from build123d import *

# Parameters (mm, degrees)
F2_W      = 22
F2_H      = 45.6
F2_R      = 1.7
F3_DEPTH  = 4
F4_R      = 5
F5_R      = 3.99999
F6_DEPTH  = 3
F8_R      = 9
F9_DEPTH  = 12
F10_R     = 2.85
F11_DEPTH = 8
F12_R     = 2.15
F13_DEPTH = 8
F13_TAPER = -0.5
F14_SIZE2 = 4
F14_SIZE  = 2


# Not quite as in the source:
# - a fillet or chamfer is up to 0.001 mm smaller than in the source, because OpenCascade refuses the exact size
# - a feature names something its author has since deleted; it is built from what else it names


with BuildPart() as f3:
    # F2 (on Top) → F3 (new body)
    with BuildSketch(Plane.XY):
        Rectangle(F2_W, F2_H)
        Polygon((3.3486315613, -16.9), (1.6743157806, -19.8), (-1.6743157806, -19.8), (-3.3486315613, -16.9), (-1.6743157806, -14), (1.6743157806, -14), align=None, mode=Mode.SUBTRACT)
        Circle(F2_R, mode=Mode.SUBTRACT)
        Polygon((1.6743157806, 19.8), (3.3486315613, 16.9), (1.6743157806, 14), (-1.6743157806, 14), (-3.3486315613, 16.9), (-1.6743157806, 19.8), align=None, mode=Mode.SUBTRACT)
        Polygon((1.6743157806, 14), (3.3486315613, 16.9), (1.6743157806, 19.8), (-1.6743157806, 19.8), (-3.3486315613, 16.9), (-1.6743157806, 14), align=None)
        with Locations((0, 16.9)):
            Circle(F2_R, mode=Mode.SUBTRACT)
        Circle(F2_R)
        Polygon((-1.6743157806, -19.8), (1.6743157806, -19.8), (3.3486315613, -16.9), (1.6743157806, -14), (-1.6743157806, -14), (-3.3486315613, -16.9), align=None)
        with Locations((0, -16.9)):
            Circle(F2_R, mode=Mode.SUBTRACT)
    extrude(amount=-F3_DEPTH)

    # F4
    f4_edges = [f3.edges().sort_by_distance(p)[0] for p in [
        (-11, 22.8, -2),
        (11, 22.8, -2),
        (11, -22.8, -2),
        (-11, -22.8, -2),
    ]]
    fillet(f4_edges, radius=F4_R)

    # F5 (radius 4 in the source; OpenCascade refuses exactly that, so slightly less here)
    f5_edges = [f3.edges().sort_by_distance(p)[0] for p in [
        (-11, 0, 0),
        (0, -22.8, 0),
        (-9.535534, -21.335534, 0),
        (9.535534, -21.335534, 0),
        (11, 0, 0),
        (9.535534, 21.335534, 0),
        (0, 22.8, 0),
        (-9.535534, 21.335534, 0),
    ]]
    fillet(f5_edges, radius=F5_R)

    # F2 (on Top) → F6 (cut)
    with BuildSketch(Plane.XY):
        Polygon((1.6743157806, 14), (3.3486315613, 16.9), (1.6743157806, 19.8), (-1.6743157806, 19.8), (-3.3486315613, 16.9), (-1.6743157806, 14), align=None)
        with Locations((0, 16.9)):
            Circle(F2_R, mode=Mode.SUBTRACT)
        Polygon((-1.6743157806, -19.8), (1.6743157806, -19.8), (3.3486315613, -16.9), (1.6743157806, -14), (-1.6743157806, -14), (-3.3486315613, -16.9), align=None)
        with Locations((0, -16.9)):
            Circle(F2_R, mode=Mode.SUBTRACT)
    extrude(amount=-F6_DEPTH, mode=Mode.SUBTRACT)

    # F8 (on line) → F9 (join)
    with BuildSketch(Plane.XY):
        Circle(F8_R)
    extrude(amount=F9_DEPTH)

    # F10 (on face) → F11 (cut)
    with BuildSketch(Plane.XY.offset(12)):
        Circle(F10_R)
    extrude(amount=-F11_DEPTH, mode=Mode.SUBTRACT)

    # F12 (on face) → F13 (cut, through all)
    with BuildSketch(Plane.XY.offset(4)):
        Circle(F12_R)
    extrude(amount=-F13_DEPTH, taper=F13_TAPER, mode=Mode.SUBTRACT)

    # F14
    f14_edges = [f3.edges().sort_by_distance(p)[0] for p in [
        (-9, 0, 12),
    ]]
    f14_side = f3.faces().sort_by_distance((-8.745442, 0, 12))[0]
    chamfer(f14_edges, length=F14_SIZE, length2=F14_SIZE2, reference=f14_side)


solid = f3.part
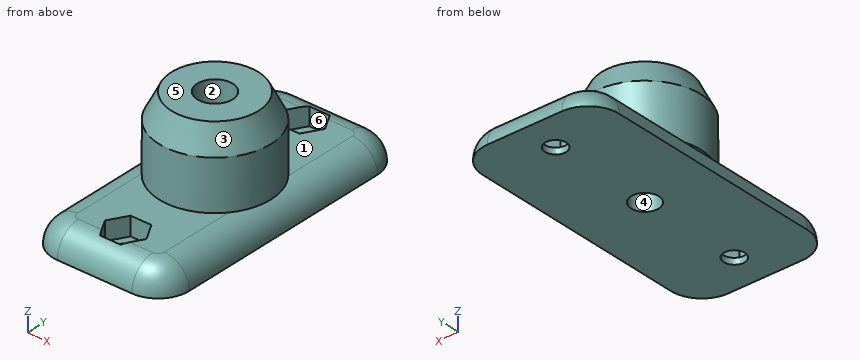
Design review of the part built by this model. Coordinates are the model's own, in mm. Face numbers are marked on the shaded views. A direction names the side the tool comes from. Round coordinates to 2 decimals unless told otherwise and drop trailing zeros. Write each loop counter-clockwise with the first axis right and the second up, starting at its lowest first coordinate (ties: lowest second). Pieces come first, ordered by that corner, then holes. Notation, with made-up numbers: M 29,7 L 46,7 A23 ccw 46,32 Z; hole C -29,42.5 d11. An arc over 180 degrees is marked long. One line per item, written item: value. Start each with the question number.
1. For the marked faces 4, 5 and 6, list the 3-axis set-ups (+Z, -Z, +X, -X, +Y, -Y) from which the entire face can be reached by the end or side of a thin tool; tool diameter is ignored.
2. Take a section at B-B on z = 5. State the section outline as (x, y) points.
3. To check wall thickness, follow probe 1 along Y at (x, z) = (0, -3.5); probe 2 along Y at (x, z) = (0.25, 6); probe 3 along Y at (x, z) = (0, -3.25). State the ranges of each line that lie inside material, in increasing order. Write a range as from..to.
4. Draft analysis for pull direction X (two halves, no side actions). For the marked faces 1, 2 and 3, state which applies: pulls with the +X half, pulls with the -X half, needs draft (parallel to the pull), parting line crosses it, or undercut.
5. Take a section at D-D on z = 2.75. State the section outline as (x, y) points.
6. Take a section at A-A on x = 0. State how many separate pieces and enclosed holes the cut face has, then the cut area to 3 significant figures.
7. Clearance check with flat-ended pins moving along their axes: P1, Ø1.5, axis at x = -1, z = -1.5, coming from the -Y side; P2, Ø5, axis at x = -7, z = 6.5, coming from the +Y side; P3, Ø1.4, axis at x = 0.5, z = -1.5, coming from the +Y side. State where each tip first meets the part, or that it passes through.
Computed:
1. face 4: -Z
1. face 5: +Z, +X, -X, +Y, -Y
1. face 6: +Z
2. outline: C 0,0 d18; hole C 0,0 d5.7
3. probe 1: y = -22.77..-18.6, -15.2..-2.22, 2.22..15.2, 18.6..22.77
3. probe 2: y = -9..-2.84, 2.84..9
3. probe 3: y = -22.73..-18.6, -15.2..-2.21, 2.21..15.2, 18.6..22.73
4. face 1: needs draft
4. face 2: undercut
4. face 3: parting line crosses it
5. outline: C 0,0 d18; hole C 0,0 d4.32
6. separate pieces: 4
6. enclosed holes: 0
6. area: 261 mm²
7. P1: stops at y = -22.4
7. P2: stops at y = 7.79
7. P3: stops at y = 22.37
